Input: part model. Units: mm. Frame: model coordinates. Face numbers are marked on the shaded views. A direction names the side the tool comes from. Give positions to 0.01 mm unless a question says otherwise; leave off trailing zeros. Loops run counter-clockwise (first coordinate to the right, second up) from the corner with the lowest first, then second, coordinate; pieces in that order, holes last. Notation, with made-up numbers: (21.5, 74) - (38.5, 74) arc R15 ccw to (38.5, 95) - close; hole circle Ø6 at (-11, -12.75). An arc over 180 degrees is marked (long way). Answer as a JSON object with one key per item and string values. Group by question number.
(1) Material intervals for L1, parallel to X at y = 1, z = -40; L2, parallel to Z at x = 15, y = 3.05; L3, parallel to X at y = 170, z = -49.5, sorted ascending.
(2) Section query C-C (y = 146). Return loops of the section in (x, z), plus the area to 3 significant figures.
(3) Pin query (flat end, axial travel): P1, Ø12, axis at y = 144.5, z = -189, coming from the +X side; P2, Ø1, axis at y = 34, z = -39.5, coming from the -X side; P3, Ø5, axis at x = 106, y = 72.5, coming from the -Z side. Return the tip coordinate at first contact, or that it passes through.
(4) Section query B-B (z = -184). Return loops of the section in (x, y), plus the area to 3 significant figures.
(5) Access query for the marked faces 4, 5 and 6. Directions: +Z, -Z, +X, -X, +Y, -Y. A direction counts if a zero-diameter tool reaches every point of the face in a straight line with its end or side. Return the directions, or none.
(6) Mould query, pull axis Y, two halves, no side actions, for the marked faces 1, 2 and 3. Classes: +Y half, -Y half, draft (parallel to the pull), parting line (faces both ways), or undercut.
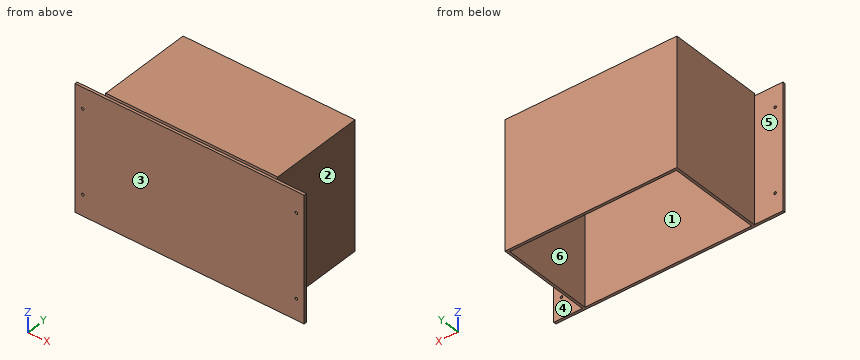
Autodesk Inventor part; units mm, degrees
ref_plane "YZ Plane" through (0, 0, 0) normal (1, 0, 0) x (0, 1, 0)
ref_plane "XZ Plane" through (0, 0, 0) normal (0, 1, 0) x (-1, 0, 0)
ref_plane "XY Plane" through (0, 0, 0) normal (0, 0, 1) x (1, 0, 0)
sketch "Sketch1" plane through (0, 0, 0) normal (0, 0, 1) x (1, 0, 0)
  line L0 (0, 0) -> (440, 0)
  line L1 (220, 0) -> (380, 0)
  line L2 (220, 0) -> (60, 0)
  line L3 (60, 2.9881) -> (60, 182.9881)
  line L4 (60, 182.9881) -> (380, 182.9881)
  line L5 (380, 182.9881) -> (380, 0)
  line L6 (60, -5) -> (220, -5)
  line L7 (220, -5) -> (385, -5)
  line L8 (385, -5) -> (385, 187.9881)
  line L9 (385, 187.9881) -> (55, 187.9881)
  line L10 (55, 187.9881) -> (55, 2.9881)
  line L11 (0, 0) -> (0, 5)
  line L12 (0, 5) -> (440, 5)
  line L13 (440, 5) -> (440, 0)
  point P0 (385, 5)
  point P1 (55, 5)
  point P2 (380, 5)
  point P3 (60, 5)
  dimension "d0" = 440
  dimension "d1" = 160
  dimension "d2" = 160
  dimension "d3" = 180
  dimension "d4" = 5
  dimension "d5" = 5
extrude "Extrusion1" add sketch "Sketch1" against normal blind 240 contours L11 L12 L5 L0 | L10 L9 L8 L12 L5 L4 L3 | L5 L12 L8 L0 | L8 L12 L13 L0
sketch "Sketch2" plane through (0, 5, 0) normal (0, 1, 0) x (1, 0, 0)
  line L0 (0, 0) -> (0, 240)
  line L1 (0, 240) -> (15, 240)
  line L2 (440, 240) -> (0, 240)
  line L3 (15, 240) -> (15, -108.1496)
  line L4 (440, 240) -> (425, 240)
  line L5 (425, 240) -> (425, -108.1496)
  circle A0 centre (15, 200) radius 2.5
  circle A1 centre (15, 40) radius 2.5
  line L6 (55, 0) -> (0, 0)
  line L7 (220, 240) -> (220, -68.5309)
  circle A2 centre (425, 200) radius 2.5
  circle A3 centre (425, 40) radius 2.5
  dimension "d8" = 15
  dimension "d9" = 15
  dimension "d10" = 5
  dimension "d11" = 5
  dimension "d12" = 40
  dimension "d13" = 40
extrude "Extrusion2" cut sketch "Sketch2" against normal blind 215 contours A3 L5 | L5 A3 | A2 L5 | L5 A2 | A1 L3 | L3 A1 | A0 L3 | L3 A0
sketch "Sketch3" plane through (0, 0, 0) normal (0, 0, 1) x (1, 0, 0)
  line L0 (0, 5) -> (55, 5)
  line L1 (55, 187.9881) -> (385, 187.9881)
  line L2 (55, 5) -> (385, 5)
  line L3 (385, 5) -> (385, 187.9881)
  line L4 (385, 187.9881) -> (55, 187.9881)
  line L5 (55, 187.9881) -> (55, 5)
  point P0 (60, 5)
  point P1 (380, 182.9881)
extrude "Extrusion3" add sketch "Sketch3" along normal blind 5
properties part number "Proteção de acrilico-Painel de controle"
Recorded:
{
 "1": {"L1": "x = 0 to 12.5, 17.5 to 422.5, 427.5 to 440", "L2": "z = -240 to -202.5, -197.5 to -42.5, -37.5 to 0", "L3": "x = 55 to 60, 380 to 385"},
 "2": {"outline": "(55, -240) - (60, -240) - (60, 0) - (380, 0) - (380, -240) - (385, -240) - (385, 5) - (55, 5) - close", "area": "4,050 mm^2"},
 "3": {"P1": "stops at x = 385", "P2": "stops at x = 55", "P3": "stops at z = 0"},
 "4": {"outline": "(0, 0) - (440, 0) - (440, 5) - (385, 5) - (385, 187.99) - (55, 187.99) - (55, 5) - (0, 5) - close; hole (60, 5) - (380, 5) - (380, 182.99) - (60, 182.99) - close", "area": "5,630 mm^2"},
 "5": {"face 4": "+Z, -Z, +X, +Y", "face 5": "+Z, -Z, -X, +Y", "face 6": "-Z"},
 "6": {"face 1": "undercut", "face 2": "draft", "face 3": "-Y half"}
}
